Here's how the part is built. I have some questions about the finished solid (model axes, mm). A direction names the side the tool comes from. Give positions to 0.01 mm unless a question says otherwise; leave off trailing zeros. Write each loop counter-clockwise with the first axis right and the second up, starting at its lowest first coordinate (ties: lowest second). Pieces come first, ordered by that corner, then holes. Notation, with made-up numbers: (50.25, 82) -> (98.25, 82) arc R17 cw to (98.25, 86) -> close; hole circle Ø2 at (-20.5, -3.75). An arc over 180 degrees is marked (long way). Return JSON: item names as keys, results as strings.
from build123d import *

# Parameters (mm, degrees)
SKETCH1_R           = 1
BOSS_EXTRUDE1_DEPTH = 5
SKETCH3_W           = 51
SKETCH3_H           = 56
BOSS_EXTRUDE3_DEPTH = 2
SKETCH7_W           = 70
SKETCH7_H           = 100
SKETCH7_R           = 1.5
BOSS_EXTRUDE5_DEPTH = 2


with BuildPart() as part:
    # Sketch1 → Boss-Extrude1 (new body)
    with BuildSketch(Plane.XY):
        Polygon((-25.5, -13), (25.5, -13), (25.5, 13), (25.5, 17), (25.5, 43), (-25.5, 43), (-25.5, 17), (-25.5, 13), align=None)
        with Locations((-23.500000003, 11.000000003)):
            Circle(SKETCH1_R, mode=Mode.SUBTRACT)
        with Locations((-23.500000003, -11.000000003)):
            Circle(SKETCH1_R, mode=Mode.SUBTRACT)
        with Locations((23.500000003, -11.000000003)):
            Circle(SKETCH1_R, mode=Mode.SUBTRACT)
        with Locations((23.500000003, 11.000000003)):
            Circle(SKETCH1_R, mode=Mode.SUBTRACT)
        with Locations((23.500000003, 18.999999997)):
            Circle(SKETCH1_R, mode=Mode.SUBTRACT)
        with Locations((23.500000003, 41.000000003)):
            Circle(SKETCH1_R, mode=Mode.SUBTRACT)
        with Locations((-23.500000003, 41.000000003)):
            Circle(SKETCH1_R, mode=Mode.SUBTRACT)
        with Locations((-23.500000003, 18.999999997)):
            Circle(SKETCH1_R, mode=Mode.SUBTRACT)
    extrude(amount=BOSS_EXTRUDE1_DEPTH)

    # Sketch3 → Boss-Extrude3 (add)
    with BuildSketch(Plane.XY.offset(5)):
        with Locations((0, 15)):
            Rectangle(SKETCH3_W, SKETCH3_H)
    extrude(amount=BOSS_EXTRUDE3_DEPTH)

    # Sketch7 → Boss-Extrude5 (add)
    with BuildSketch(Plane.XY.offset(7)):
        with Locations((0, 15)):
            Rectangle(SKETCH7_W, SKETCH7_H)
        with Locations((-25.5, -30)):
            Circle(SKETCH7_R, mode=Mode.SUBTRACT)
        with Locations((25.5, -30)):
            Circle(SKETCH7_R, mode=Mode.SUBTRACT)
        with Locations((25.5, 60)):
            Circle(SKETCH7_R, mode=Mode.SUBTRACT)
        with Locations((-25.5, 60)):
            Circle(SKETCH7_R, mode=Mode.SUBTRACT)
    extrude(amount=BOSS_EXTRUDE5_DEPTH)


solid = part.part
1. If I drill on line 1 (Y direction, x = 25.5, z = 8.45); line 2 (X direction, y = 19, z = 2); line 3 (Y direction, x = -23.5, z = 1.9), over which ranges is the centre line in solid material (lowest first)? Write a range as [from, to].
Taken from the geometry:
{"line 1": "y = [-35, -31.5], [-28.5, 58.5], [61.5, 65]", "line 2": "x = [-25.5, -24.5], [-22.5, 22.5], [24.5, 25.5]", "line 3": "y = [-13, -12], [-10, 10], [12, 18], [20, 40], [42, 43]"}
2. For pin 1 Ø1 at (x, y) = (23.5, 11) entering from -Z; pin 2 Ø1 at (x, z) = (-8, 1) entering from -Y; pin 3 Ø3 at (y, z) = (13, 2) entering from +X, each with a flat end and sliding along its axis, tell me the tip position at first contact or that it passes through.
Taken from the geometry:
{"pin 1": "stops at z = 5", "pin 2": "stops at y = -13", "pin 3": "stops at x = 25.5"}
3. Suppose I cut it at D-D, the plane x = 29.5. List the corners of the cut face in (y, z) for me.
Taken from the geometry:
{"outline": "(-35, 7) -> (65, 7) -> (65, 9) -> (-35, 9) -> close"}
4. Which directions (+Z, -Z, +X, -X, +Y, -Y) give clear straight access to the entire face, cutting with the end or side of a thin tool? Please do faces 4 (the face through (-24, 11, 5)), 5 (the face through (-25.5, 15, 3)), 6 (the face through (0, 43, 3)).
Taken from the geometry:
{"face 4": "-Z", "face 5": "-Z, -X, +Y, -Y", "face 6": "-Z, +X, -X, +Y"}
5. Suppose I cut it at C-C, the plane y = -1.5. List the corners of the cut face in (x, z) for me.
Taken from the geometry:
{"outline": "(-35, 7) -> (-25.5, 7) -> (-25.5, 0) -> (25.5, 0) -> (25.5, 7) -> (35, 7) -> (35, 9) -> (-35, 9) -> close"}
6. Suppose I cut it at B-B, the plane x = 9. List the corners of the cut face in (y, z) for me.
Taken from the geometry:
{"outline": "(-35, 7) -> (-13, 7) -> (-13, 0) -> (43, 0) -> (43, 7) -> (65, 7) -> (65, 9) -> (-35, 9) -> close"}
7. Suppose I cut it at A-A, the plane y = 11. List the corners of the cut face in (x, z) for me.
Taken from the geometry:
{"outline": "(-35, 7) -> (-25.5, 7) -> (-25.5, 0) -> (-24.5, 0) -> (-24.5, 5) -> (-22.5, 5) -> (-22.5, 0) -> (22.5, 0) -> (22.5, 5) -> (24.5, 5) -> (24.5, 0) -> (25.5, 0) -> (25.5, 7) -> (35, 7) -> (35, 9) -> (-35, 9) -> close"}
8. If we mould it in two halves opening along X, with no side actions, what happens to faces 1 (the face through (-24, -11, 5)), 2 (the face through (25.5, 15, 3)), 3 (the face through (0, -13, 3))? For each: released by +X, released by -X, zero draft, split by the parting line, or undercut.
Taken from the geometry:
{"face 1": "undercut", "face 2": "released by +X", "face 3": "zero draft"}
